```python
from build123d import *

# Parameters (mm, degrees)
SKETCH_R      = 1.5
PAD_DEPTH     = 1
SKETCH001_W   = 10
SKETCH001_H   = 10
SKETCH001_W_2 = 4.857736
SKETCH001_H_2 = 4.857736
SKETCH001_W_3 = 5.662197
SKETCH001_H_3 = 7.409003
SKETCH001_H_4 = 4.857737
PAD001_DEPTH  = 2


with BuildPart() as part:
    # Sketch → Pad (new body)
    with BuildSketch(Plane.XY):
        with BuildLine():
            Line((-17.25, 19), (17.25, 19))
            ThreePointArc((19, 17.25), (18.487437, 18.487437), (17.25, 19))
            Line((19, 17.25), (19, -17.25))
            ThreePointArc((17.25, -19), (18.487437, -18.487437), (19, -17.25))
            Line((17.25, -19), (-17.25, -19))
            ThreePointArc((-19, -17.25), (-18.487437, -18.487437), (-17.25, -19))
            Line((-19, -17.25), (-19, 17.25))
            ThreePointArc((-17.25, 19), (-18.487437, 18.487437), (-19, 17.25))
        make_face()
        with Locations((15.25, 15.25)):
            Circle(SKETCH_R, mode=Mode.SUBTRACT)
        with Locations((-15.25, -15.25)):
            Circle(SKETCH_R, mode=Mode.SUBTRACT)
        with Locations((-15.25, 15.25)):
            Circle(SKETCH_R, mode=Mode.SUBTRACT)
        with Locations((15.25, -15.25)):
            Circle(SKETCH_R, mode=Mode.SUBTRACT)
    extrude(amount=PAD_DEPTH)

    # Sketch001 (on Face14 of Pad) → Pad001 (join)
    with BuildSketch(Plane.XY.offset(1)):
        with Locations((0.198833, -6.963992)):
            Rectangle(SKETCH001_W, SKETCH001_H)
        with Locations((-9.179753, 15.701071)):
            Rectangle(SKETCH001_W_2, SKETCH001_H_2)
        with Locations((0.053276, 7.817709)):
            Rectangle(SKETCH001_W_3, SKETCH001_H_3)
        with Locations((-9.179753, 9.504914)):
            Rectangle(SKETCH001_W_2, SKETCH001_H_4)
        with Locations((-9.179753, 3.308758)):
            Rectangle(SKETCH001_W_2, SKETCH001_H_4)
        with Locations((-9.179753, -2.887397)):
            Rectangle(SKETCH001_W_2, SKETCH001_H_4)
        with Locations((-9.179753, -9.083554)):
            Rectangle(SKETCH001_W_2, SKETCH001_H_2)
        with Locations((-9.179753, -15.27971)):
            Rectangle(SKETCH001_W_2, SKETCH001_H_2)
        with Locations((9.179753, 15.701071)):
            Rectangle(SKETCH001_W_2, SKETCH001_H_2)
        with Locations((9.179753, 9.504914)):
            Rectangle(SKETCH001_W_2, SKETCH001_H_4)
        with Locations((9.179753, 3.308758)):
            Rectangle(SKETCH001_W_2, SKETCH001_H_4)
        with Locations((9.179753, -2.887397)):
            Rectangle(SKETCH001_W_2, SKETCH001_H_4)
        with Locations((9.179753, -9.083554)):
            Rectangle(SKETCH001_W_2, SKETCH001_H_2)
        with Locations((9.179753, -15.27971)):
            Rectangle(SKETCH001_W_2, SKETCH001_H_2)
    extrude(amount=PAD001_DEPTH)


solid = part.part
```
Input: part model. Units: mm. Frame: model coordinates. A direction names the side the tool comes from. Coordinates: 2 decimals unless noted, no trailing zeros. Order: outer loops, then holes, each group sorted by start corner. A loop starts at its lowest first (then second) coordinate and runs counter-clockwise, first axis right, second up. Notation, with made-up numbers: (-11, 84) - (-1, 84) arc R15 ccw to (-1, 90) - close; hole circle Ø5 at (-32.75, 11.25). An arc over 180 degrees is marked (long way). Return JSON: item names as keys, results as strings.
Q1. Access query for faces 5 (the flat face through (-9, -12.851, 2)), 6 (the flat face through (-11.609, 9, 2)), 7 (the flat face through (5.199, -7, 2)). Directions: +Z, -Z, +X, -X, +Y, -Y. A direction counts if a zero-diameter tool reaches every point of the face in a straight line with its end or side. Return the directions, or none.
The answers:
{"face 5": "+Z, +X, -X", "face 6": "+Z, -X, +Y, -Y", "face 7": "+Z, +Y, -Y"}
Q2. Cut plane B-B (x = 15.25). Return loops of the section in (y, z).
The answers:
{"outline": "(-19, 0) - (-16.75, 0) - (-16.75, 1) - (-19, 1) - close; (-13.75, 0) - (13.75, 0) - (13.75, 1) - (-13.75, 1) - close; (16.75, 0) - (19, 0) - (19, 1) - (16.75, 1) - close"}
Q3. Ray query, probe 1 along Y at (x, z) = (-15.25, 0.25); probe 2 along X at (y, z) = (4.5, 2.3); probe 3 along Y at (x, z) = (-11, 2.45). Return the intervals inside material, ascending.
The answers:
{"probe 1": "y = -19 to -16.75, -13.75 to 13.75, 16.75 to 19", "probe 2": "x = -11.61 to -6.75, -2.78 to 2.88, 6.75 to 11.61", "probe 3": "y = -17.71 to -12.85, -11.51 to -6.65, -5.32 to -0.46, 0.88 to 5.74, 7.08 to 11.93, 13.27 to 18.13"}
Q4. Cut plane C-C (z = 0.55). Return loops of the section in (x, y).
The answers:
{"outline": "(-19, -17.25) arc R1.75 ccw to (-17.25, -19) - (17.25, -19) arc R1.75 ccw to (19, -17.25) - (19, 17.25) arc R1.75 ccw to (17.25, 19) - (-17.25, 19) arc R1.75 ccw to (-19, 17.25) - close; hole circle Ø3 at (-15.25, -15.25); hole circle Ø3 at (-15.25, 15.25); hole circle Ø3 at (15.25, -15.25); hole circle Ø3 at (15.25, 15.25)"}
Q5. Cut plane A-A (y = 15.25). Return loops of the section in (x, z), then the cut area to 3 significant figures.
The answers:
{"outline": "(-19, 0) - (-16.75, 0) - (-16.75, 1) - (-19, 1) - close; (-13.75, 0) - (13.75, 0) - (13.75, 1) - (11.61, 1) - (11.61, 3) - (6.75, 3) - (6.75, 1) - (-6.75, 1) - (-6.75, 3) - (-11.61, 3) - (-11.61, 1) - (-13.75, 1) - close; (16.75, 0) - (19, 0) - (19, 1) - (16.75, 1) - close", "area": "51.4 mm2"}
Q6. Cut plane D-D (x = -10). Return loops of the section in (y, z), then the cut area to 3 significant figures.
The answers:
{"outline": "(-19, 0) - (19, 0) - (19, 1) - (18.13, 1) - (18.13, 3) - (13.27, 3) - (13.27, 1) - (11.93, 1) - (11.93, 3) - (7.08, 3) - (7.08, 1) - (5.74, 1) - (5.74, 3) - (0.88, 3) - (0.88, 1) - (-0.46, 1) - (-0.46, 3) - (-5.32, 3) - (-5.32, 1) - (-6.65, 1) - (-6.65, 3) - (-11.51, 3) - (-11.51, 1) - (-12.85, 1) - (-12.85, 3) - (-17.71, 3) - (-17.71, 1) - (-19, 1) - close", "area": "96.3 mm2"}
Q7. Draft query along Y for faces 1 (the flat face through (11.609, -3, 2)), 2 (the flat face through (9, -17.709, 2)), 3 (the flat face through (9, 13.272, 2)), 4 (the cylindrical face through (-18.474, 18.501, 0.493)). Return one class per face: +Y half, -Y half, draft (parallel to the pull), parting line (faces both ways), or undercut.
The answers:
{"face 1": "draft", "face 2": "-Y half", "face 3": "undercut", "face 4": "+Y half"}
Q8. First-contact query: pin 1 (1.6 mm diameter, centred on x = -1, z = 2, fed in from +Y); pin 2 (0.6 mm diameter, centred on y = -2, z = 1.5, fed in from -X); pin 3 (1 mm diameter, centred on x = 10, z = 2, fed in from -Y). Flat tips, straight axial feed; report the tip coordinate or a pass-through.
The answers:
{"pin 1": "stops at y = 11.52", "pin 2": "stops at x = -11.61", "pin 3": "stops at y = -17.71"}
